Can you work these out from the model? Positions are in its coordinate system, mm. Face numbers are marked on the shaded views. A direction names the side the tool comes from. Give positions to 0.01 mm unless a question says otherwise; leave off trailing zeros. Loops run counter-clockwise (first coordinate to the right, second up) from the corner with the lowest first, then second, coordinate; pieces in that order, holes last.
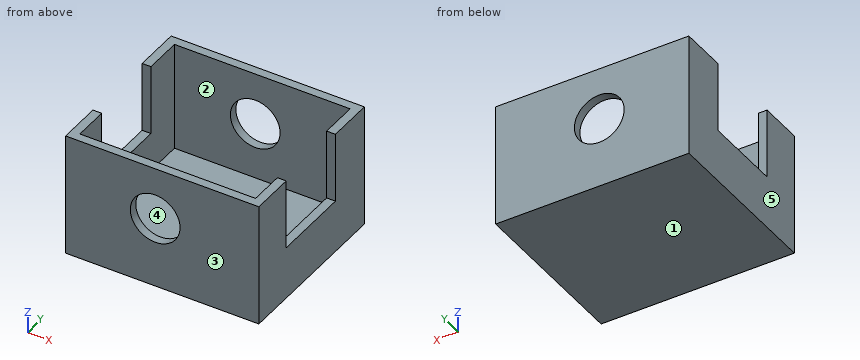
from build123d import *

# Parameters (mm, degrees)
F0_W      = 110
F0_H      = 70
F1_DEPTH  = 8
F2_W      = 5
F2_H      = 40
F2_H_2    = 25
F3_DEPTH  = 62.1
F4_W      = 28
F4_H      = 40
F5_DEPTH  = 117.8
F7_DEPTH  = 15.5
F8_DEPTH  = 17
F9_R      = 14.1609686348
F10_DEPTH = 96.5309327604


with BuildPart() as f1:
    # F0 (on Top) → F1 (new body)
    with BuildSketch(Plane.XY):
        with Locations((4.0090922266, 13.2649663802)):
            Rectangle(F0_W, F0_H)
    extrude(amount=F1_DEPTH)

    # F2 (on face) → F3 (join)
    with BuildSketch(Plane.XY.offset(8)):
        Polygon((59.0090922266, 48.2649663802), (-50.9909077734, 48.2649663802), (-50.9909077734, 43.2649663802), (-45.9909077734, 43.2649663802), (54.0090922266, 43.2649663802), (59.0090922266, 43.2649663802), align=None)
        with Locations((-48.4909077734, 23.2649663802)):
            Rectangle(F2_W, F2_H)
        with Locations((56.5090922266, 23.2649663802)):
            Rectangle(F2_W, F2_H)
        with Locations((-48.4909077734, -9.2350336198)):
            Rectangle(F2_W, F2_H_2)
        with Locations((56.5090922266, -9.2350336198)):
            Rectangle(F2_W, F2_H_2)
    extrude(amount=F3_DEPTH)

    # F4 (on face) → F5 (cut)
    with BuildSketch(Plane(origin=(-50.9909077734, 0, 0), x_dir=(0, -1, 0), z_dir=(-1, 0, 0))):
        with Locations((7.7350336198, 50.1)):
            Rectangle(F4_W, F4_H)
    extrude(amount=-F5_DEPTH, mode=Mode.SUBTRACT)

    # F6: F1 across plane


with BuildPart() as f1_1:
    add(f1.part)
    add(f1.part.mirror(Plane.XZ))

    # F7 (cut): faces of the model
    f7_faces = [f1_1.faces().sort_by_distance(p)[0] for p in [
        (-48.4909077734, 6.2649663802, 50.1),
        (56.5090922266, 6.2649663802, 50.1),
    ]]
    extrude(f7_faces, amount=-F7_DEPTH, mode=Mode.SUBTRACT)

    # F8 (cut): faces of the model
    f8_faces = [f1_1.faces().sort_by_distance(p)[0] for p in [
        (56.5090922266, -6.2649663802, 50.1),
        (-48.4909077734, -6.2649663802, 50.1),
    ]]
    extrude(f8_faces, amount=-F8_DEPTH, mode=Mode.SUBTRACT)

    # F9 (on face) → F10 (cut, through all)
    with BuildSketch(Plane(origin=(0, 48.2649663802, 0), x_dir=(-1, 0, 0), z_dir=(0, 1, 0))):
        with Locations((0, 40.3115488589)):
            Circle(F9_R)
    extrude(amount=-F10_DEPTH, mode=Mode.SUBTRACT)


solid = f1_1.part
(1) Suppose I cut it at D-D on z = 19. List the corners of the cut face in (x, y) for me, plus the area to 3 significant figures.
Returned:
outline: (-50.99, -48.26) - (59.01, -48.26) - (59.01, 48.26) - (-50.99, 48.26) - close; hole (-45.99, -43.26) - (54.01, -43.26) - (54.01, 43.26) - (-45.99, 43.26) - close
area: 1,970 mm2
(2) Thinking about a two-plate mould opening in X: for the marked faces 3, 4 and 5, which applies, pulls with the +X half, pulls with the -X half, needs draft (parallel to the pull), parting line crosses it, or undercut?
Returned:
face 3: needs draft
face 4: undercut
face 5: pulls with the -X half
(3) Please list where these lines run through material, in increasing order: probe 1 along X at (y, z) = (-11, 22); probe 2 along Y at (x, z) = (5.5, 57.5); probe 3 along Z at (x, y) = (0, -46.25).
Returned:
probe 1: x = -50.99 to -45.99, 54.01 to 59.01
probe 2: y = -48.26 to -43.26, 43.26 to 48.26
probe 3: z = 0 to 26.15, 54.47 to 70.1
(4) Suppose I cut it at A-A on z = 62. List the corners of the cut face in (x, y) for me.
Returned:
outline: (-50.99, -48.26) - (59.01, -48.26) - (59.01, -23.26) - (54.01, -23.26) - (54.01, -43.26) - (-45.99, -43.26) - (-45.99, -23.26) - (-50.99, -23.26) - close; (-50.99, 21.76) - (-45.99, 21.76) - (-45.99, 43.26) - (54.01, 43.26) - (54.01, 21.76) - (59.01, 21.76) - (59.01, 48.26) - (-50.99, 48.26) - close
(5) Suppose I cut it at C-C on y = -2. List the corners of the cut face in (x, z) for me, plus the area to 3 significant figures.
Returned:
outline: (-50.99, 0) - (59.01, 0) - (59.01, 30.1) - (54.01, 30.1) - (54.01, 8) - (-45.99, 8) - (-45.99, 30.1) - (-50.99, 30.1) - close
area: 1,100 mm2
(6) Which directions (+Z, -Z, +X, -X, +Y, -Y) give clear straight access to the entire face, cutting with the end or side of a thin tool? Please do the marked faces 1 and 2.
Returned:
face 1: -Z, +X, -X, +Y, -Y
face 2: +Z
(7) Will these pins go through, and if not, where does the flat tip stop? P1, Ø4, axis at x = 57, y = -4, coming from the +Z side; P2, Ø5, axis at y = -22, z = 59.5, coming from the +X side; P3, Ø1, axis at x = 14.5, y = 28.5, coming from the +Z side.
Returned:
P1: stops at z = 30.1
P2: stops at x = 59.01
P3: stops at z = 8
(8) Suppose I cut it at B-B on x = 0. List the corners of the cut face in (y, z) for me, plus the area to 3 significant figures.
Returned:
outline: (-48.26, 0) - (48.26, 0) - (48.26, 26.15) - (43.26, 26.15) - (43.26, 8) - (-43.26, 8) - (-43.26, 26.15) - (-48.26, 26.15) - close; (-48.26, 54.47) - (-43.26, 54.47) - (-43.26, 70.1) - (-48.26, 70.1) - close; (43.26, 54.47) - (48.26, 54.47) - (48.26, 70.1) - (43.26, 70.1) - close
area: 1,110 mm2
